For this review, use the dimensioned drawing (mm, ordinates from the lowest corner) and the shaded views. Coordinates: 2 decimals unless noted, no trailing zeros. Order: outer loops, then holes, each group sorted by start corner. A loop starts at its lowest first (then second) coordinate and runs counter-clockwise, first axis right, second up. Notation, with made-up numbers: M 54.5,45.25 L 86.5,45.25 A22 cw 86.5,60.25 Z; hole C 31,-34 d8. An arc over 180 degrees is marked long. One line per item, written item: value.
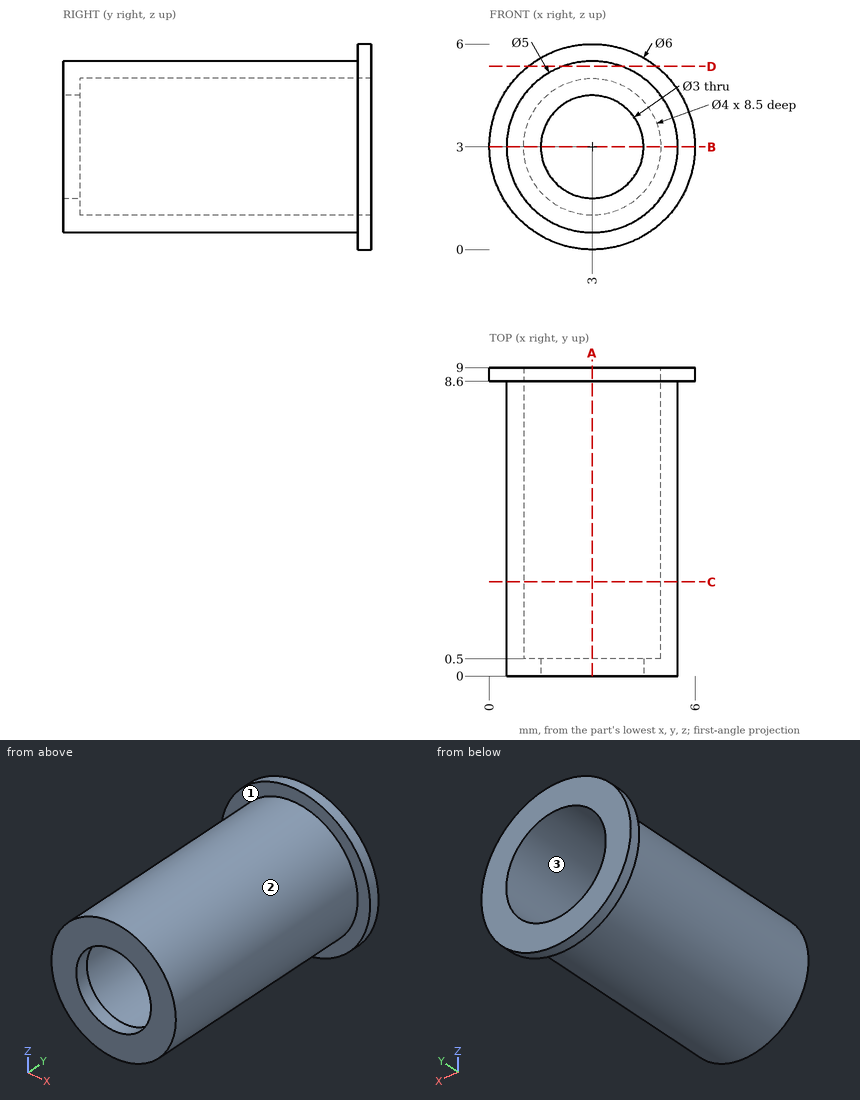
(1) For L1, parallel to X at y = 6.5, z = 3; L2, parallel to X at y = 0.3, z = 3; L3, parallel to Y at x = 4.95, z = 3.25, list the stretches that pass through material, from the lowest coordinate up.
Geometry results:
L1: x = 0.5 to 1, 5 to 5.5
L2: x = 0.5 to 1.5, 4.5 to 5.5
L3: y = 0 to 0.5
(2) We need section C-C, the plane y = 2.75. State the section outline as (x, z) points, plus the area to 3 significant figures.
Geometry results:
outline: C 3,3 d5; hole C 3,3 d4
area: 7.07 mm2
(3) Insertion check: pin 1 Ø1.5 at (y, z) = (1.5, 5) entering from -X. The pin has a flat end and moves straight along its axis. Give the tip position at first contact, or say it passes through.
Geometry results:
pin 1: stops at x = 0.83
(4) We need section A-A, the plane x = 3. State the section outline as (y, z) points, plus the area to 3 significant figures.
Geometry results:
outline: M 0,0.5 L 8.6,0.5 L 8.6,0 L 9,0 L 9,1 L 0.5,1 L 0.5,1.5 L 0,1.5 Z; M 0,4.5 L 0.5,4.5 L 0.5,5 L 9,5 L 9,6 L 8.6,6 L 8.6,5.5 L 0,5.5 Z
area: 9.90 mm2
(5) We need section B-B, the plane z = 3. State the section outline as (x, y) points, plus the area to 3 significant figures.
Geometry results:
outline: M 0,8.6 L 0.5,8.6 L 0.5,0 L 1.5,0 L 1.5,0.5 L 1,0.5 L 1,9 L 0,9 Z; M 4.5,0 L 5.5,0 L 5.5,8.6 L 6,8.6 L 6,9 L 5,9 L 5,0.5 L 4.5,0.5 Z
area: 9.90 mm2
(6) Mouldability with a two-part tool opening along X and no side actions: class the marked faces 1, 2 and 3 as +X half, -X half, draft (parallel to the pull), parting line (faces both ways), or undercut.
Geometry results:
face 1: draft
face 2: parting line
face 3: undercut
(7) We need section D-D, the plane z = 5.35. State the section outline as (x, y) points, plus the area to 3 significant figures.
Geometry results:
outline: M 1.14,8.6 L 2.15,8.6 L 2.15,0 L 3.85,0 L 3.85,8.6 L 4.86,8.6 L 4.86,9 L 1.14,9 Z
area: 16.2 mm2
